from build123d import *

# Parameters (mm, degrees)
SKETCH_1_R          = 1.6
SKETCH_1_R_2        = 8
EXTRUDE_1_DEPTH     = 3
SKETCH_2_R          = 9.5
CUT_EXTRUDE_1_DEPTH = 10


with BuildPart() as part:
    # 草图1 → 凸台-拉伸1 (new body)
    with BuildSketch(Plane.XY):
        with BuildLine():
            Line((27.996813697, 12.530864127), (49.744946635, -38.957900319))
            Line((49.744946635, -38.957900319), (-28.813781546, -38.957900319))
            Line((-28.813781546, -38.957900319), (-34.369737997, 8.111506623))
            ThreePointArc((-34.369737997, 8.111506623), (-22.106553261, 32.655394345), (5.290025786, 31.166911584))
            Line((5.290025786, 31.166911584), (22.752678609, 19.002490435))
            ThreePointArc((22.752678609, 19.002490435), (25.832973998, 16.137991786), (27.996813697, 12.530864127))
        make_face()
        with Locations((-19.091881546, 20.591881546)):
            Circle(SKETCH_1_R, mode=Mode.SUBTRACT)
        with Locations((-19.09157413, 1.492010657)):
            Circle(SKETCH_1_R, mode=Mode.SUBTRACT)
        with Locations((0, 1.5)):
            Circle(SKETCH_1_R, mode=Mode.SUBTRACT)
        with Locations((0.000307159, 20.583891946)):
            Circle(SKETCH_1_R, mode=Mode.SUBTRACT)
        with Locations((-9.542099681, 11.042099681)):
            Circle(SKETCH_1_R_2, mode=Mode.SUBTRACT)
        with Locations((10.457900319, -14.042678355)):
            Circle(SKETCH_1_R, mode=Mode.SUBTRACT)
        with Locations((30.457900319, -29.042678355)):
            Circle(SKETCH_1_R, mode=Mode.SUBTRACT)
        with Locations((-9.542099681, -29.042678355)):
            Circle(SKETCH_1_R, mode=Mode.SUBTRACT)
        with Locations((23.762798875, 11.821649257)):
            Circle(SKETCH_1_R, mode=Mode.SUBTRACT)
        with Locations((12.088647332, 9.044206953)):
            Circle(SKETCH_1_R, mode=Mode.SUBTRACT)
    extrude(amount=EXTRUDE_1_DEPTH)

    # 草图2 → 切除-拉伸1 (cut)
    with BuildSketch(Plane.XY.offset(3)):
        with Locations((-9.542099681, 11.042099681)):
            Circle(SKETCH_2_R)
    extrude(amount=-CUT_EXTRUDE_1_DEPTH, mode=Mode.SUBTRACT)


solid = part.part
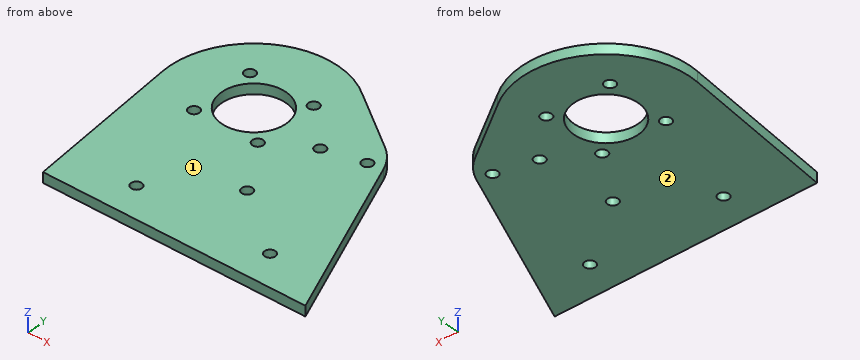
Check sheet for the modelled part. Datum: model origin and axes. Units: mm. Face numbers are marked on the shaded views. Give positions to 0.01 mm unless a question says otherwise; leave off trailing zeros. Write each loop counter-clockwise with the first axis right and the second up, starting at its lowest first coordinate (ties: lowest second). Pieces come first, ordered by that corner, then holes. Notation, with made-up numbers: (55.5, 24) -> (94.5, 24) arc R24 ccw to (94.5, 60) -> close; hole circle Ø8 at (16.25, -23). An arc over 180 degrees is marked (long way). One line per item, written item: value. Start each with the question number.
Item 1: Section check D-D on x = 4. Record the cut outline in (y, z).
Item 2: Section check A-A on x = -15.5. Record the cut outline in (y, z), then the cut area to 3 significant figures.
Item 3: Gauge pin test, flat ends, axial feed: pin 1 (5 mm diameter, centred on x = 10.46, y = -14.04, fed in from -Z); pin 2 (1 mm diameter, centred on y = 4, z = 2, fed in from -X). Record the tip position at first contact, or that the pin passes through.
Item 4: Draft check along Z on the marked faces 1 and 2. Enter one of: +Z half, -Z half, draft (parallel to the pull), parting line (faces both ways), or undercut.
Item 5: Material ranges on probe 1 along X at (y, z) = (10.5, 0.9); probe 2 along Y at (x, z) = (-5.5, 2.3); probe 3 along X at (y, z) = (21, 2.85), recorded low to high. Write a range as from..to.
Item 6: Section check C-C on y = -6. Record the cut outline in (x, z), then the cut area to 3 significant figures.
Item 7: Section check B-B on z = 2.35. State how many separate pieces and enclosed holes the cut face has, then the cut area to 3 significant figures.
Results list:
1. outline: (-38.96, 0) -> (32.06, 0) -> (32.06, 3) -> (-38.96, 3) -> close
2. outline: (-38.96, 0) -> (3.64, 0) -> (3.64, 3) -> (-38.96, 3) -> close; (18.44, 0) -> (35.32, 0) -> (35.32, 3) -> (18.44, 3) -> close
2. area: 178 mm²
3. pin 1: z = 0
3. pin 2: x = -33.94
4. face 1: +Z half
4. face 2: -Z half
5. probe 1: -34.54..-19.03, -0.06..11.42, 12.75..22.86, 24.66..28.85
5. probe 2: -38.96..2.44, 19.64..35.71
5. probe 3: -32.47..-20.64, -17.54..-1.54, 1.55..19.89
6. outline: (-32.7, 0) -> (35.82, 0) -> (35.82, 3) -> (-32.7, 3) -> close
6. area: 206 mm²
7. separate pieces: 1
7. enclosed holes: 10
7. area: 4,300 mm²
